Geometry: final body of the model. Coordinates: model frame, mm. A direction names the side the tool comes from. Round coordinates to 2 decimals unless told otherwise and drop trailing zeros. Write each loop counter-clockwise with the first axis right and the second up, starting at its lowest first coordinate (ties: lowest second). Pieces come first, ordered by that corner, then holes. Notation, with made-up numbers: (89.25, 41.25) - (98.25, 41.25) arc R33 ccw to (98.25, 78.25) - close; hole circle Ø9 at (29, -10). An arc over 180 degrees is marked (long way). Write each question's results on one line, items separated by ' | '.
from build123d import *

# Parameters (mm, degrees)
SQUARE_TUBE_CONFIGURED_2_X_2_X_0_25_1_DEPTH = 285.75
CUT_EXTRUDE1_DEPTH                          = 218.733740656
CUT_EXTRUDE1_DEPTH_BACK                     = 218.733740656


with BuildPart() as part:
    # Sketch11 → Square tube - configured 2 X 2 X 0.25(1) (new body)
    with BuildSketch(Plane.YZ.offset(-68.758290896)):
        with BuildLine():
            Line((-10.16, -12.7), (10.16, -12.7))
            ThreePointArc((10.16, -12.7), (11.956051224, -11.956051224), (12.7, -10.16))
            Line((12.7, -10.16), (12.7, 10.16))
            ThreePointArc((12.7, 10.16), (11.956051224, 11.956051224), (10.16, 12.7))
            Line((10.16, 12.7), (-10.16, 12.7))
            ThreePointArc((-10.16, 12.7), (-11.956051224, 11.956051224), (-12.7, 10.16))
            Line((-12.7, 10.16), (-12.7, -10.16))
            ThreePointArc((-12.7, -10.16), (-11.956051224, -11.956051224), (-10.16, -12.7))
        make_face()
        with BuildLine():
            Line((-10.16, -10.287), (10.16, -10.287))
            ThreePointArc((10.16, -10.287), (10.249802561, -10.249802561), (10.287, -10.16))
            Line((10.287, -10.16), (10.287, 10.16))
            ThreePointArc((10.287, 10.16), (10.249802561, 10.249802561), (10.16, 10.287))
            Line((10.16, 10.287), (-10.16, 10.287))
            ThreePointArc((-10.16, 10.287), (-10.249802561, 10.249802561), (-10.287, 10.16))
            Line((-10.287, 10.16), (-10.287, -10.16))
            ThreePointArc((-10.287, -10.16), (-10.249802561, -10.249802561), (-10.16, -10.287))
        make_face(mode=Mode.SUBTRACT)
    extrude(amount=SQUARE_TUBE_CONFIGURED_2_X_2_X_0_25_1_DEPTH)

    # Sketch12 → Cut-Extrude1 (cut, two sides: drawn at the far end of the back side and taken through both)
    with BuildSketch(Plane.XY.offset(-CUT_EXTRUDE1_DEPTH_BACK)):
        Polygon((-68.758290896, -12.7), (-43.358290896, 12.7), (-68.758290896, 12.7), align=None)
        Polygon((216.991709104, -12.7), (191.591709104, 12.7), (216.991709104, 12.7), align=None)
    extrude(amount=CUT_EXTRUDE1_DEPTH + CUT_EXTRUDE1_DEPTH_BACK, mode=Mode.SUBTRACT)


solid = part.part
Q1. Access query for faces 1 (the flat face through (72, -10.287, 0)), 2 (the flat face through (72, -12.7, 0)). Directions: +Z, -Z, +X, -X, +Y, -Y. A direction counts if a zero-diameter tool reaches every point of the face in a straight line with its end or side. Return the directions, or none.
Answer block:
face 1: +X, -X | face 2: +Z, -Z, +X, -X, -Y
Q2. Section query B-B, the plane x = -11.5. Return loops of the section in (y, z).
Answer block:
outline: (-12.7, -10.16) arc R2.54 ccw to (-10.16, -12.7) - (10.16, -12.7) arc R2.54 ccw to (12.7, -10.16) - (12.7, 10.16) arc R2.54 ccw to (10.16, 12.7) - (-10.16, 12.7) arc R2.54 ccw to (-12.7, 10.16) - close; hole (-10.29, -10.16) arc R0.13 ccw to (-10.16, -10.29) - (10.16, -10.29) arc R0.13 ccw to (10.29, -10.16) - (10.29, 10.16) arc R0.13 ccw to (10.16, 10.29) - (-10.16, 10.29) arc R0.13 ccw to (-10.29, 10.16) - close
Q3. Section query C-C, the plane y = -5. Return loops of the section in (x, z).
Answer block:
outline: (-61.06, -12.7) - (209.29, -12.7) - (209.29, -10.29) - (-61.06, -10.29) - close; (-61.06, 10.29) - (209.29, 10.29) - (209.29, 12.7) - (-61.06, 12.7) - close
Q4. Section query A-A, the plane z = 2.25. Return loops of the section in (x, y), plus the area to 3 significant figures.
Answer block:
outline: (-68.76, -12.7) - (216.99, -12.7) - (214.58, -10.29) - (-66.35, -10.29) - close; (-45.77, 10.29) - (194, 10.29) - (191.59, 12.7) - (-43.36, 12.7) - close | area: 1,260 mm2
Q5. Mould query, pull axis Z, two halves, no side actions, for faces 3 (the flat face through (204.47, -0.18, 11.11)), 4 (the flat face through (72, 0, -12.7)), 5 (the flat face through (72, 0, -10.287)). Classes: pulls with the +Z half, pulls with the -Z half, needs draft (parallel to the pull), parting line crosses it, or undercut.
Answer block:
face 3: needs draft | face 4: pulls with the -Z half | face 5: undercut
Q6. Ray query, line 1 along Z through (x, y) = (-41, 2); line 2 along Z through (x, y) = (89, -10.5). Return the intervals inside material, ascending.
Answer block:
line 1: -12.7 to -10.29, 10.29 to 12.7 | line 2: -12.68 to 12.68
